```python
from build123d import *

# Parameters (mm, degrees)
SKETCH1_R                                           = 39.37
BOSS_EXTRUDE1_DEPTH                                 = 9.525
SKETCH2_R                                           = 38.1
BOSS_EXTRUDE2_DEPTH                                 = 603.25
SHELL1_T                                            = -2.54
CSK_FOR_5_16_FLAT_HEAD_MACHINE_SCREW_10_D           = 8.4328
CSK_FOR_5_16_FLAT_HEAD_MACHINE_SCREW_10_DEPTH       = 12.7
CSK_FOR_5_16_FLAT_HEAD_MACHINE_SCREW_10_CSINK_D     = 16.129
CSK_FOR_5_16_FLAT_HEAD_MACHINE_SCREW_10_CSINK_ANGLE = 100
CSK_FOR_5_16_FLAT_HEAD_MACHINE_SCREW_10_TIP         = 2.533468714


with BuildPart() as part:
    # Sketch1 → Boss-Extrude1 (new body)
    with BuildSketch(Plane(origin=(0, 0, 0), x_dir=(1, 0, 0), z_dir=(0, 1, 0))):
        with Locations(Location((0, 0, 0), (0, 0, 90))):
            Circle(SKETCH1_R)
    extrude(amount=BOSS_EXTRUDE1_DEPTH)

    # Sketch2 → Boss-Extrude2 (add)
    with BuildSketch(Plane(origin=(0, 9.525, 0), x_dir=(1, 0, 0), z_dir=(0, 1, 0))):
        with Locations(Location((0, 0, 0), (0, 0, 270))):
            Circle(SKETCH2_R)
    extrude(amount=BOSS_EXTRUDE2_DEPTH)

    # Shell1
    shell1_openings = [part.faces().sort_by_distance(p)[0] for p in [
        (0, 0, 0),
    ]]
    offset(amount=SHELL1_T, openings=shell1_openings, kind=Kind.INTERSECTION)

    # Sketch4 → Revolve1 (revolve)
    with BuildSketch(Plane.XY, mode=Mode.PRIVATE) as revolve1_sk:
        Polygon((0, 612.775), (30.48, 612.775), (30.48, 617.855), (31.75, 619.125), (31.75, 635.635), (29.21, 638.175), (0, 638.175), align=None)
    revolve(revolve1_sk.sketch.rotate(Axis((0, 0, 0), (0, 1, 0)), 90), axis=Axis((0, 0, 0), (0, 1, 0)))

    # CSK for 5/16 Flat Head Machine Screw (100)1
    with Locations(Plane(origin=(0, 638.175, 0), x_dir=(1, 0, 0), z_dir=(0, 1, 0))):
        with Locations((0, 0)):
            CounterSinkHole(CSK_FOR_5_16_FLAT_HEAD_MACHINE_SCREW_10_D / 2, CSK_FOR_5_16_FLAT_HEAD_MACHINE_SCREW_10_CSINK_D / 2, depth=CSK_FOR_5_16_FLAT_HEAD_MACHINE_SCREW_10_DEPTH, counter_sink_angle=CSK_FOR_5_16_FLAT_HEAD_MACHINE_SCREW_10_CSINK_ANGLE)
            with Locations((0, 0, -(CSK_FOR_5_16_FLAT_HEAD_MACHINE_SCREW_10_DEPTH + CSK_FOR_5_16_FLAT_HEAD_MACHINE_SCREW_10_TIP / 2))):  # 118° drill point
                Cone(0, CSK_FOR_5_16_FLAT_HEAD_MACHINE_SCREW_10_D / 2, CSK_FOR_5_16_FLAT_HEAD_MACHINE_SCREW_10_TIP, mode=Mode.SUBTRACT)


solid = part.part
```
Geometry check sheet. Reference: the model listing, model coordinates, mm. A direction names the side the tool comes from. Coordinates: 2 decimals unless noted, no trailing zeros. Order: outer loops, then holes, each group sorted by start corner. A loop starts at its lowest first (then second) coordinate and runs counter-clockwise, first axis right, second up. Notation, with made-up numbers: (1, -14.5) - (32, -14.5) arc R29 cw to (32, 19.5) - close; hole circle Ø9 at (-28.5, 55). An arc over 180 degrees is marked (long way). Answer in a Markdown table with one row per item. Add a question column.
1. Draft check along X on faces 5 (the face through (-30.22, 615.35, 3.97)), 6 (the face through (3.245, 635.103, -2.976)), 7 (the face through (-21, 9.525, 32)). Enter one of: +X half, -X half, draft (parallel to the pull), parting line (faces both ways), or undercut.
2. Material ranges on L1, parallel to X at y = 348, z = 0; L2, parallel to X at y = 1.75, z = 0; L3, parallel to Y at x = 9, z = -36 (3 decimals), recorded low to high. Write a range as [from, to].
3. Gauge pin test, flat ends, axial feed: pin 1 Ø10 at (x, z) = (-4.5, 14) entering from -Y (3 decimals); pin 2 Ø3 at (y, z) = (462.5, 12) entering from -X; pin 3 Ø2 at (y, z) = (439, 31) entering from -X. Record the tip position at first contact, or that the pin passes through.
4. Access from +Z, -Z, +X, -X, +Y, -Y to the whole of each face (thin tool, end or side, straight path). Record for faces 1 (the face through (29, 0, -23)), 2 (the face through (-34.714, 304.387, -7.709)), 3 (the face through (-23.183, 306.927, -30.235)), 4 (the face through (26, 612.775, -17)).
5. Section check A-A (y = 537). Enter the section's corners in (x, z).
Data:
| question | item | result |
|---|---|---|
| 1 | face 5 | parting line |
| 1 | face 6 | undercut |
| 1 | face 7 | draft |
| 2 | L1 | x = [-38.1, -35.56], [35.56, 38.1] |
| 2 | L2 | x = [-39.37, -36.83], [36.83, 39.37] |
| 2 | L3 | y = [0, 612.775] |
| 3 | pin 1 | stops at y = 610.235 |
| 3 | pin 2 | stops at x = -36.62 |
| 3 | pin 3 | stops at x = -23.49 |
| 4 | face 1 | +Z, -Z, +X, -X, -Y |
| 4 | face 2 | -Y |
| 4 | face 3 | +Y |
| 4 | face 4 | none |
| 5 | outline | circle Ø76.2 at (0, 0); hole circle Ø71.12 at (0, 0) |
